Geometry: final body of the model. Coordinates: model frame, mm. Face numbers are marked on the shaded views. A direction names the side the tool comes from. Coordinates: 2 decimals unless noted, no trailing zeros. Loops run counter-clockwise (first coordinate to the right, second up) from the corner with the lowest first, then second, coordinate; pieces in that order, holes last. Notation, with made-up numbers: (13, -25.5) - (38, -25.5) arc R22 cw to (38, -18.5) - close; hole circle Ø5 at (-2, -6.5). An arc over 180 degrees is marked (long way). Answer in a Markdown table with one row per item.
from build123d import *

# Parameters (mm, degrees)
SKETCH1_R           = 1.4
BOSS_EXTRUDE1_DEPTH = 18.7
SKETCH2_R           = 0.95
BOSS_EXTRUDE2_DEPTH = 9.1
SKETCH3_R           = 1.85
BOSS_EXTRUDE3_DEPTH = 1.7
SKETCH4_R           = 1.4
BOSS_EXTRUDE4_DEPTH = 3.2
BOSS_EXTRUDE5_DEPTH = 28.3
SKETCH7_W           = 11.3
SKETCH7_H           = 22.6
BOSS_EXTRUDE6_DEPTH = 25.3


with BuildPart() as part:
    # Sketch1 → Boss-Extrude1 (new body)
    with BuildSketch(Plane(origin=(0, 0, 0), x_dir=(1, 0, 0), z_dir=(0, 1, 0))):
        with BuildLine():
            Line((-25.3, 11.15), (9, 11.15))
            ThreePointArc((9, 11.15), (10.414213562, 10.564213562), (11, 9.15))
            Line((11, 9.15), (11, -9.15))
            ThreePointArc((11, -9.15), (10.414213562, -10.564213562), (9, -11.15))
            Line((9, -11.15), (-25.3, -11.15))
            Line((-25.3, -11.15), (-25.3, 11.15))
        make_face()
        with Locations(Location((-20.1, 8.75, 0), (0, 0, 270))):
            Circle(SKETCH1_R, mode=Mode.SUBTRACT)
        with Locations(Location((-20.1, -8.75, 0), (0, 0, 270))):
            Circle(SKETCH1_R, mode=Mode.SUBTRACT)
    extrude(amount=BOSS_EXTRUDE1_DEPTH)

    # Sketch2 → Boss-Extrude2 (add)
    with BuildSketch(Plane(origin=(0, 18.7, 0), x_dir=(1, 0, 0), z_dir=(0, 1, 0))):
        with BuildLine():
            ThreePointArc((1.85, 2.034698995), (0, 2.75), (-1.85, 2.034698995))
            Line((-1.85, 2.034698995), (-1.85, -2.034698995))
            ThreePointArc((-1.85, -2.034698995), (0, -2.75), (1.85, -2.034698995))
            Line((1.85, -2.034698995), (1.85, 2.034698995))
        make_face()
        with Locations(Location((0, 0, 0), (0, 0, 270))):
            Circle(SKETCH2_R, mode=Mode.SUBTRACT)
    extrude(amount=BOSS_EXTRUDE2_DEPTH)

    # Sketch3 → Boss-Extrude3 (add)
    with BuildSketch(Plane(origin=(0, 18.7, 0), x_dir=(1, 0, 0), z_dir=(0, 1, 0))):
        with Locations(Location((-11.2, 0, 0), (0, 0, 270))):
            Circle(SKETCH3_R)
    extrude(amount=BOSS_EXTRUDE3_DEPTH)

    # Sketch4 → Boss-Extrude4 (add)
    with BuildSketch(Plane(origin=(0, 7.2, 0), x_dir=(-1, 0, 0), z_dir=(0, -1, 0))):
        with BuildLine():
            Line((-11, -2.95), (-15, -2.95))
            ThreePointArc((-15, -2.95), (-15.707106781, -2.657106781), (-16, -1.95))
            Line((-16, -1.95), (-16, 1.95))
            ThreePointArc((-16, 1.95), (-15.707106781, 2.657106781), (-15, 2.95))
            Line((-15, 2.95), (-11, 2.95))
            Line((-11, 2.95), (-11, -2.95))
        make_face()
        with Locations(Location((-13.4, 0, 0), (0, 0, 90))):
            Circle(SKETCH4_R, mode=Mode.SUBTRACT)
    extrude(amount=-BOSS_EXTRUDE4_DEPTH)

    # Sketch5 → Boss-Extrude5 (add)
    with BuildSketch(Plane.ZY.offset(25.3)):
        with BuildLine():
            Line((-2.6, 17.1), (2.6, 17.1))
            ThreePointArc((2.6, 17.1), (11.15, 8.55), (2.6, 0))
            Line((2.6, 0), (-2.6, 0))
            ThreePointArc((-2.6, 0), (-11.15, 8.55), (-2.6, 17.1))
        make_face()
    extrude(amount=BOSS_EXTRUDE5_DEPTH)

    # Sketch7 → Boss-Extrude6 (add)
    with BuildSketch(Plane.ZY.offset(53.6)):
        with Locations((0, 8.55)):
            Rectangle(SKETCH7_W, SKETCH7_H)
    extrude(amount=-BOSS_EXTRUDE6_DEPTH)


solid = part.part
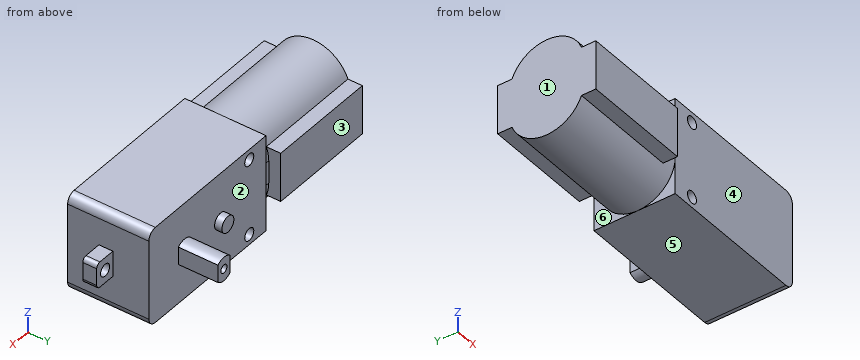
(1) Pull-direction query (X, two-part tool) for the marked faces 1, 2 and 3; classes: pulls with the +X half, pulls with the -X half, needs draft (parallel to the pull), parting line crosses it, or undercut.
Verdict:
| item | result |
|---|---|
| face 1 | pulls with the -X half |
| face 2 | undercut |
| face 3 | needs draft |
(2) Cut plane D-D on z = -8.25. Output: boundary loops of the cut face in (x, y).
Verdict:
| item | result |
|---|---|
| outline | (-53.6, 2.13) - (-25.3, 2.13) - (-25.3, 0) - (-21.41, 0) - (-21.41, 18.7) - (-25.3, 18.7) - (-25.3, 14.97) - (-53.6, 14.97) - close; (-18.79, 0) - (11, 0) - (11, 18.7) - (-18.79, 18.7) - close |
(3) Cut plane A-A on x = 13.4. Output: boundary loops of the cut face in (y, z), then the cut area to 3 significant figures.
Verdict:
| item | result |
|---|---|
| outline | (7.2, -2.95) - (10.4, -2.95) - (10.4, -1.4) - (7.2, -1.4) - close; (7.2, 1.4) - (10.4, 1.4) - (10.4, 2.95) - (7.2, 2.95) - close |
| area | 9.92 mm² |
(4) Access query for the marked faces 4, 5 and 6. Directions: +Z, -Z, +X, -X, +Y, -Y. A direction counts if a zero-diameter tool reaches every point of the face in a straight line with its end or side. Return the directions, or none.
Verdict:
| item | result |
|---|---|
| face 4 | +Z, -Z, +X, -Y |
| face 5 | -Z, +X, -X, +Y, -Y |
| face 6 | +Y |
(5) Cut plane B-B on y = 2.5. Output: boundary loops of the cut face in (x, z), then the cut area to 3 significant figures.
Verdict:
| item | result |
|---|---|
| outline | (-53.6, -8.64) - (-25.3, -8.64) - (-25.3, -11.15) - (9, -11.15) arc R2 ccw to (11, -9.15) - (11, 9.15) arc R2 ccw to (9, 11.15) - (-25.3, 11.15) - (-25.3, 8.64) - (-53.6, 8.64) - close; hole circle Ø2.8 at (-20.1, -8.75); hole circle Ø2.8 at (-20.1, 8.75) |
| area | 1,280 mm² |
(6) Cut plane C-C on x = -11.2. Output: boundary loops of the cut face in (y, z), then the cut area to 3 significant figures.
Verdict:
| item | result |
|---|---|
| outline | (0, -11.15) - (18.7, -11.15) - (18.7, -1.85) - (20.4, -1.85) - (20.4, 1.85) - (18.7, 1.85) - (18.7, 11.15) - (0, 11.15) - close |
| area | 423 mm² |
(7) Ray query, probe 1 along X at (y, z) = (9.5, 0); probe 2 along Y at (x, z) = (8, 10.25); probe 3 along Z at (x, y) = (-42, 17.5). Return the intervals inside material, ascending.
Verdict:
| item | result |
|---|---|
| probe 1 | x = -53.6 to 12, 14.8 to 16 |
| probe 2 | y = 0 to 18.7 |
| probe 3 | z = -5.65 to 5.65 |
(8) First-contact query: pin 1 Ø2 at (x, y) = (-41.5, 13) entering from -Z; pin 2 Ø2.5 at (x, z) = (13.5, 1.5) entering from -Y; pin 3 Ø2.5 at (x, z) = (-27, 0.5) entering from +Y. Flat tips, straight axial feed; report the tip coordinate or a pass-through.
Verdict:
| item | result |
|---|---|
| pin 1 | stops at z = -10.42 |
| pin 2 | stops at y = 7.2 |
| pin 3 | stops at y = 17.1 |
